from build123d import *

# Parameters (mm, degrees)
BOSS_EXTRUDE3_DEPTH = 100
BOSS_EXTRUDE4_DEPTH = 3
BOSS_EXTRUDE5_DEPTH = 3


with BuildPart() as part:
    # Sketch1 → Boss-Extrude3 (new body)
    with BuildSketch(Plane(origin=(0, 0, 0), x_dir=(0, 1, 0), z_dir=(0, 0, 1))):
        with BuildLine():
            Line((7, 0), (139.441461344, 0))
            ThreePointArc((139.441461344, 0), (144.391208812, 2.050252532), (146.441461344, 7))
            Line((146.441461344, 7), (146.441461344, 69))
            ThreePointArc((146.441461344, 69), (144.391208812, 73.949747468), (139.441461344, 76))
            Line((139.441461344, 76), (7, 76))
            ThreePointArc((7, 76), (2.050252532, 73.949747468), (0, 69))
            Line((0, 69), (0, 7))
            ThreePointArc((0, 7), (2.050252532, 2.050252532), (7, 0))
        make_face()
        with BuildLine():
            Line((3, 38), (3, 67.481223709))
            ThreePointArc((3, 67.481223709), (4.757359313, 71.723864396), (9, 73.481223709))
            Line((9, 73.481223709), (137, 73.481223709))
            ThreePointArc((137, 73.481223709), (141.242640687, 71.723864396), (143, 67.481223709))
            Line((143, 67.481223709), (143, 9.481223709))
            ThreePointArc((143, 9.481223709), (141.242640687, 5.238583022), (137, 3.481223709))
            Line((137, 3.481223709), (9, 3.481223709))
            ThreePointArc((9, 3.481223709), (4.757359313, 5.238583022), (3, 9.481223709))
            Line((3, 9.481223709), (3, 38))
        make_face(mode=Mode.SUBTRACT)
    extrude(amount=BOSS_EXTRUDE3_DEPTH)

    # Sketch1<5> → Boss-Extrude4 (add)
    with BuildSketch(Plane(origin=(0, 0, 0), x_dir=(0, 1, 0), z_dir=(0, 0, 1))):
        with BuildLine():
            Line((151, 38), (151, 6))
            ThreePointArc((151, 6), (147.778174593, -1.778174593), (140, -5))
            Line((140, -5), (6, -5))
            ThreePointArc((6, -5), (-1.778174593, -1.778174593), (-5, 6))
            Line((-5, 6), (-5, 70))
            ThreePointArc((-5, 70), (-1.778174593, 77.778174593), (6, 81))
            Line((6, 81), (73.220730672, 81))
            Line((73.220730672, 81), (140, 81))
            ThreePointArc((140, 81), (147.778174593, 77.778174593), (151, 70))
            Line((151, 70), (151, 38))
        make_face()
    extrude(amount=-BOSS_EXTRUDE4_DEPTH)

    # Sketch2 → Boss-Extrude5 (add)
    with BuildSketch(Plane.XY.offset(100)):
        with BuildLine():
            Line((-70, 151), (-6, 151))
            ThreePointArc((-6, 151), (1.778174593, 147.778174593), (5, 140))
            Line((5, 140), (5, 6))
            ThreePointArc((5, 6), (1.778174593, -1.778174593), (-6, -5))
            Line((-6, -5), (-70, -5))
            ThreePointArc((-70, -5), (-77.778174593, -1.778174593), (-81, 6))
            Line((-81, 6), (-81, 140))
            ThreePointArc((-81, 140), (-77.778174593, 147.778174593), (-70, 151))
        make_face()
        with BuildLine():
            Line((-67.481223709, 143), (-9.481223709, 143))
            ThreePointArc((-9.481223709, 143), (-5.238583022, 141.242640687), (-3.481223709, 137))
            Line((-3.481223709, 137), (-3.481223709, 9))
            ThreePointArc((-3.481223709, 9), (-5.238583022, 4.757359313), (-9.481223709, 3))
            Line((-9.481223709, 3), (-67.481223709, 3))
            ThreePointArc((-67.481223709, 3), (-71.723864396, 4.757359313), (-73.481223709, 9))
            Line((-73.481223709, 9), (-73.481223709, 137))
            ThreePointArc((-73.481223709, 137), (-71.723864396, 141.242640687), (-67.481223709, 143))
        make_face(mode=Mode.SUBTRACT)
    extrude(amount=BOSS_EXTRUDE5_DEPTH)


solid = part.part
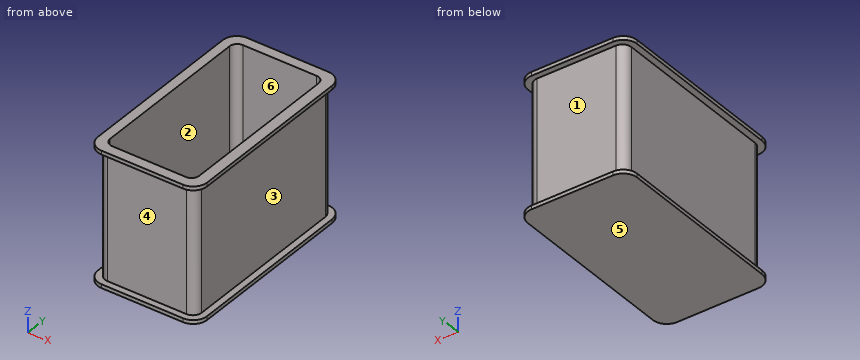
Here's how the part is built. I have some questions about the finished solid (model axes, mm). Face numbers are marked on the shaded views. A direction names the side the tool comes from. Coordinates: 2 decimals unless noted, no trailing zeros. Write each loop counter-clockwise with the first axis right and the second up, starting at its lowest first coordinate (ties: lowest second). Pieces come first, ordered by that corner, then holes. Notation, with made-up numbers: (-37, 28) - (-6, 28) arc R21 ccw to (-6, 49) - close; hole circle Ø3 at (5.5, -2). An arc over 180 degrees is marked (long way). Use one line per item in the form item = value.
1) I need wall thicknesses on line 1 (X direction, y = 93, z = 38); line 2 (Y direction, x = -49.5, z = 55); line 3 (Z direction, x = -45, y = 58). Which ranges of each line are inside material? Lowest first, please.
Solved:
line_1 = -76 to -73.48, -3.48 to 0
line_2 = 0 to 3, 143 to 146.44
line_3 = -3 to 0
2) On a 3-axis mill with a long thin cutter (end or side, diameter ignored), from which of +Z, -Z, +X, -X, +Y, -Y can I reach the whole of each face in a straight line? I mean the marked faces 1, 2 and 3. Say none if no direction works.
Solved:
face_1 = +X, -X, +Y
face_2 = +Z
face_3 = +X, +Y, -Y
3) I'm going to push flat-ended pins straight in: P1, Ø1, axis at y = 29, z = 16, coming from the +X side; P2, Ø8, axis at x = -30.5, z = 89.5, coming from the +Y side; P3, Ø4, axis at x = -37.5, y = 22, coming from the +Z side. Where does each tip first touch, or does it pass through?
Solved:
P1 = 0
P2 = 146.44
P3 = 0
4) Thinking about a two-plate mould opening in Z: for the marked faces 4, 5 and 6, which applies, released by +Z, released by -Z, zero draft, split by the parting line, or undercut?
Solved:
face_4 = undercut
face_5 = released by -Z
face_6 = zero draft
5) Suppose I cut it at A-A, the plane z = 81. Write out the boundary of the cut face in (x, y), plus the area to 3 significant figures.
Solved:
outline = (-76, 7) arc R7 ccw to (-69, 0) - (-7, 0) arc R7 ccw to (0, 7) - (0, 139.44) arc R7 ccw to (-7, 146.44) - (-69, 146.44) arc R7 ccw to (-76, 139.44) - close; hole (-73.48, 9) arc R6 ccw to (-67.48, 3) - (-9.48, 3) arc R6 ccw to (-3.48, 9) - (-3.48, 137) arc R6 ccw to (-9.48, 143) - (-67.48, 143) arc R6 ccw to (-73.48, 137) - close
area = 1,320 mm2
6) Suppose I cut it at C-C, the plane x = -33. Write out the boundary of the cut face in (y, z), plus the area to 3 significant figures.
Solved:
outline = (-5, -3) - (151, -3) - (151, 0) - (146.44, 0) - (146.44, 100) - (151, 100) - (151, 103) - (143, 103) - (143, 0) - (3, 0) - (3, 103) - (-5, 103) - (-5, 100) - (0, 100) - (0, 0) - (-5, 0) - close
area = 1,160 mm2
7) Suppose I cut it at B-B, the plane y = 85. Write out the boundary of the cut face in (x, z), plus the area to 3 significant figures.
Solved:
outline = (-81, -3) - (5, -3) - (5, 0) - (0, 0) - (0, 100) - (5, 100) - (5, 103) - (-3.48, 103) - (-3.48, 0) - (-73.48, 0) - (-73.48, 103) - (-81, 103) - (-81, 100) - (-76, 100) - (-76, 0) - (-81, 0) - close
area = 906 mm2
